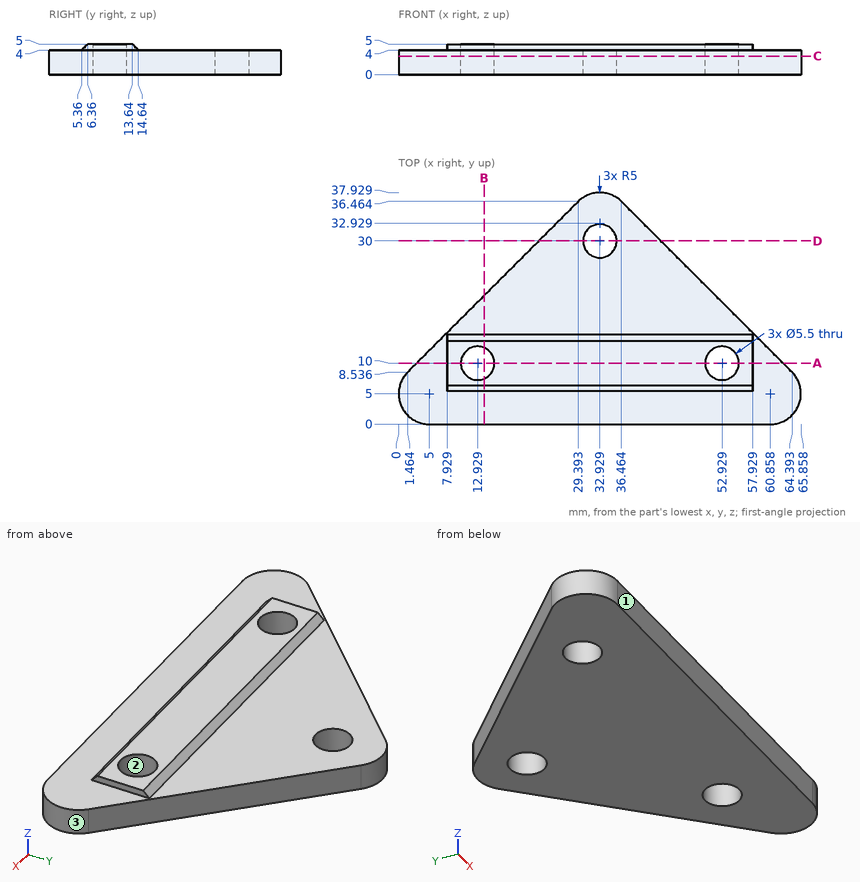
Study the drawing (mm; zero at the part's minimum x, y, z) and answer. Coordinates: 2 decimals unless noted, no trailing zeros. Write each loop counter-clockwise with the first axis right and the second up, starting at its lowest first coordinate (ties: lowest second). Pieces come first, ordered by that corner, then holes. Notation, with made-up numbers: (21, 5.5) - (63, 5.5) arc R22 ccw to (63, 31.5) - close; hole circle Ø5 at (31, -39). An arc over 180 degrees is marked (long way). One line per question, with ' | ' between items.
1) Consider probe 1 along X at (y, z) = (7.5, 1.35) (1 decimal); probe 2 along X at (y, z) = (10, 2.25); probe 3 along Z at (x, y) = (58.5, 14). Determine where each line is inside the solid, lowest interval first. Write a range as [from, to].
Checks:
probe 1: [0.7, 11.8], [14.1, 51.8], [54.1, 65.2] | probe 2: [2.93, 10.18], [15.68, 50.18], [55.68, 62.93] | probe 3: [0, 4]
2) Find section B-B, the plane x = 14. Determine the outline of the cut face in (y, z).
Checks:
outline: (0, 0) - (7.47, 0) - (7.47, 5) - (6.36, 5) - (5.36, 4) - (0, 4) - close; (12.53, 0) - (21.07, 0) - (21.07, 4) - (14.64, 4) - (13.64, 5) - (12.53, 5) - close
3) Find section C-C, the plane z = 3. Give the number of separate pieces and of enclosed holes in the cut face, and give its area (3 significant figures).
Checks:
separate pieces: 1 | enclosed holes: 3 | area: 1,460 mm2
4) Find section D-D, the plane y = 30. Determine the outline of the cut face in (x, z).
Checks:
outline: (22.93, 0) - (30.18, 0) - (30.18, 4) - (22.93, 4) - close; (35.68, 0) - (42.93, 0) - (42.93, 4) - (35.68, 4) - close
5) The mould has two halves that part along X. Classify the marked faces 1, 2 and 3: +X half, -X half, draft (parallel to the pull), parting line (faces both ways), or undercut.
Checks:
face 1: draft | face 2: undercut | face 3: +X half
6) Flat-ended cylindrical pins translate along their axes: P1, Ø9, axis at x = 32.93, y = 30, coming from the +Z side; P2, Ø0.5, axis at y = 8.5, z = 4.5, coming from the -X side. Find the tip coordinate at first contact, or state that the pin passes through.
Checks:
P1: z = 4 | P2: x = 7.93
7) Find section A-A, the plane y = 10. Determine the outline of the cut face in (x, z).
Checks:
outline: (2.93, 0) - (10.18, 0) - (10.18, 5) - (7.93, 5) - (7.93, 4) - (2.93, 4) - close; (15.68, 0) - (50.18, 0) - (50.18, 5) - (15.68, 5) - close; (55.68, 0) - (62.93, 0) - (62.93, 4) - (57.93, 4) - (57.93, 5) - (55.68, 5) - close
